from build123d import *

# Parameters (mm, degrees)
F3_R = 9.4996


# Not quite as in the source:
# - a fillet or chamfer that OpenCascade refuses, or shapes differently, is made with other operations: its cross-section is extruded or revolved along the edge and cut away or added


with BuildPart() as f1:
    # F0 (on Front) → F1 (revolve)
    with BuildSketch(Plane.XZ):
        Polygon((0, 4.7723002699), (0, 0), (64, 0), (64, 9.5), (8, 9.5), (8, 4.7723002699), align=None)
    revolve(axis=Axis((32, 0, 0), (-1, 0, 0)))

    # F2: fillet of radius 9.4996 on 1 edges, made by hand

    # F2_s1 → F2_t2 (revolve, cut)
    with BuildSketch(Plane.XZ):
        with BuildLine():
            ThreePointArc((16.2140956882, 9.5), (11.4753587068, 8.2336722524), (8, 4.7723002699))
            Line((8, 4.7723002699), (8, 9.5))
            Line((8, 9.5), (16.2140956882, 9.5))
        make_face()
    revolve(axis=Axis((8, 0, 0), (-1, 0, 0)), mode=Mode.SUBTRACT)

    # F3
    f3_edges = [f1.edges().sort_by_distance(p)[0] for p in [
        (64, 0, -9.5),
    ]]
    fillet(f3_edges, radius=F3_R)


solid = f1.part
The model under review builds one solid part; all positions refer to its coordinate system, in mm. A direction names the side the tool comes from. Give positions to 0.01 mm unless a question says otherwise; leave off trailing zeros. Loops run counter-clockwise (first coordinate to the right, second up) from the corner with the lowest first, then second, coordinate; pieces in that order, holes last. Notation, with made-up numbers: (89, -34.5) -> (138, -34.5) arc R17 ccw to (138, -1.5) -> close; hole circle Ø11 at (-25.5, -39.5). An arc over 180 degrees is marked (long way). Answer as a JSON object with one key per item and string values. Group by question number.
Q1. Wall thickness on line 1 along Y through (x, z) = (36, -0.5); line 2 along Y through (x, z) = (55.5, -8.5); line 3 along X through (y, z) = (5, 4.75): over which ranges is each line inside the solid? List them lowest first.
Q2. Insertion check: pin 1 (4 mm diameter, centred on y = 1, z = -6.5, fed in from -X); pin 2 (2 mm diameter, centred on x = 20.5, y = 2, fed in from -Z); pin 3 (6 mm diameter, centred on y = 6.5, z = 6, fed in from +X); pin 4 (1.5 mm diameter, centred on x = 38.5, z = 7.5, fed in from +Y). Each pin has a flat end and moves straight along its axis. Give the tip position at first contact, or say it passes through.
Q3. Tool access review of faces 1 (the cylindrical face through (3.94, 4.73, -0.62)), 2 (the flat face through (0, 0, 0)): name each direction out of +Z, -Z, +X, -X, +Y, -Y from which nothing blocks a thin tool from reaching the whole face with its end or side.
Q4. Take a section at A-A (x = 38.5). Write out the cut boundary in (y, z), plus the area to 3 significant figures.
Answer below:
{
 "1": {"line 1": "y = -9.49 to 9.49", "line 2": "y = -4.12 to 4.12", "line 3": "x = 9.68 to 61.03"},
 "2": {"pin 1": "stops at x = 0", "pin 2": "stops at z = -9.45", "pin 3": "stops at x = 61.99", "pin 4": "stops at y = 6.68"},
 "3": {"face 1": "-X", "face 2": "+Z, -Z, -X, +Y, -Y"},
 "4": {"outline": "circle Ø19 at (0, 0)", "area": "284 mm2"}
}
